Read the model definition and answer for the solid it produces. Units are mm, in the model's axes. A direction names the side the tool comes from. Give positions to 0.01 mm unless a question says otherwise; leave off trailing zeros. Write each loop counter-clockwise with the first axis right and the second up, starting at its lowest first coordinate (ties: lowest second). Pieces come first, ordered by that corner, then holes. Notation, with made-up numbers: M 85,-28 L 143,-28 A8 ccw 143,-15 Z; hole C 48,55.5 d8. An arc over 180 degrees is marked long. Use a Markdown table: item, result. Add a question column.
Item 1: For faces 4 (the cylindrical face through (9.734, -34.836, -23.778)), 5 (the flat face through (15.24, 3.4, -0.2)), 6 (the flat face through (9, -21, -38.1)), determine the directions among +Z, -Z, +X, -X, +Y, -Y from which every point of the face is accessible in a straight line to the end or side of a thin tool.
Item 2: A cutting plane is placed at B-B on x = 16.25. Determine the outline of the cut face in (y, z) (3 decimals).
Item 3: Consider probe 1 along Y at (x, z) = (11.5, 0) (1 decimal); probe 2 along X at (y, z) = (-37.25, -25.4); probe 3 along X at (y, z) = (8, -16.5). Determine where each line is inside the solid, lowest interval first. Write a range as [from, to].
Item 4: The mould has two halves that part along Y. Classify faces 1 (the cylindrical face through (8.652, -34.836, 23.587)), 2 (the cylindrical face through (8.77, -33.11, -0.24)), 3 (the conical face through (8.959, -27.667, -25.09)): pulls with the +Y half, pulls with the -Y half, needs draft (parallel to the pull), parting line crosses it, or undercut.
Item 5: Given P1, Ø8.5, axis at y = -1.5, z = -1.5, coming from the -X side; P2, Ø3, axis at y = 34.925, z = 0, coming from the +X side; P3, Ø10, axis at x = 12.5, z = -25, coming from the +Y side; P4, Ø15, axis at y = -4.5, z = -9.5, coming from the -X side, each flat-ended and moving along its own axis, determine where each tip first touches the part or whether it passes through.
Item 6: A cutting plane is placed at C-C on y = -31. Determine the outline of the cut face in (x, z), then the cut area to 3 significant figures.
Item 7: A cutting plane is placed at A-A on z = 0. Determine the outline of the cut face in (x, y) (1 decimal).
Item 8: A cutting plane is placed at D-D on y = -8. Determine the outline of the cut face in (x, z).
from build123d import *

# Parameters (mm, degrees)
SKETCH1_R                 = 38.1
BOSS_EXTRUDE1_DEPTH       = 17.78
SKETCH2_R                 = 25.4
CUT_EXTRUDE1_DEPTH        = 8.89
F_6_CLEARANCE_HOLE1_D     = 3.6576
SKETCH6_R                 = 14.2875
CUT_EXTRUDE2_DEPTH        = 6.35
SKETCH7_R                 = 3.175
CUT_EXTRUDE3_DEPTH        = 59.918282604
F_6_CLEARANCE_HOLE2_D     = 3.6576
F_6_CLEARANCE_HOLE2_DEPTH = 12.7
F_6_CLEARANCE_HOLE2_TIP   = 1.0988539


with BuildPart() as part:
    # Sketch1 → Boss-Extrude1 (new body)
    with BuildSketch(Plane(origin=(0, 0, 0), x_dir=(0, 0, -1), z_dir=(1, 0, 0))):
        with BuildLine():
            ThreePointArc((38.1, 0), (0, -38.1), (-38.1, 0))
            Line((-38.1, 0), (-38.1, -41.275))
            Line((-38.1, -41.275), (38.1, -41.275))
            Line((38.1, -41.275), (38.1, 0))
        make_face()
        Circle(SKETCH1_R)
    extrude(amount=BOSS_EXTRUDE1_DEPTH)

    # Sketch2 → Cut-Extrude1 (cut)
    with BuildSketch(Plane.ZY):
        Circle(SKETCH2_R)
    extrude(amount=-CUT_EXTRUDE1_DEPTH, mode=Mode.SUBTRACT)

    # #6 Clearance Hole1 (through all)
    with Locations(Plane(origin=(17.78, 0, 0), x_dir=(0, 0, -1), z_dir=(1, 0, 0))):
        with Locations((0, 34.925), (34.925, 0), (0, -34.925), (-34.925, 0)):
            Hole(F_6_CLEARANCE_HOLE1_D / 2)

    # Sketch6 → Cut-Extrude2 (cut)
    with BuildSketch(Plane.ZY.offset(-8.89)):
        Circle(SKETCH6_R)
    extrude(amount=-CUT_EXTRUDE2_DEPTH, mode=Mode.SUBTRACT)

    # Sketch7 → Cut-Extrude3 (cut, through all)
    with BuildSketch(Plane(origin=(17.78, 0, 0), x_dir=(0, 0, -1), z_dir=(1, 0, 0))):
        Circle(SKETCH7_R)
    extrude(amount=-CUT_EXTRUDE3_DEPTH, mode=Mode.SUBTRACT)

    # #6 Clearance Hole2
    with Locations(Plane(origin=(0, -41.275, 0), x_dir=(-1, 0, 0), z_dir=(0, -1, 0))):
        with Locations((-8.89, 25.4), (-8.89, -25.4)):
            Hole(F_6_CLEARANCE_HOLE2_D / 2, depth=F_6_CLEARANCE_HOLE2_DEPTH)
            with Locations((0, 0, -(F_6_CLEARANCE_HOLE2_DEPTH + F_6_CLEARANCE_HOLE2_TIP / 2))):  # 118° drill point
                Cone(0, F_6_CLEARANCE_HOLE2_D / 2, F_6_CLEARANCE_HOLE2_TIP, mode=Mode.SUBTRACT)


solid = part.part
Filled in:
| question | item | result |
|---|---|---|
| 1 | face 4 | -Y |
| 1 | face 5 | -X |
| 1 | face 6 | -Z, +X, -X, +Y, -Y |
| 2 | outline | M -41.275,-38.1 L 0,-38.1 A38.1 ccw 0,38.1 L -41.275,38.1 Z; hole C -34.925,0 d3.658; hole C 0,0 d6.35; hole C 0,-34.925 d3.658; hole C 0,34.925 d3.658; hole C 34.925,0 d3.658 |
| 3 | probe 1 | [-41.3, -36.8], [-33.1, -14.3], [14.3, 33.1], [36.8, 38.1] |
| 3 | probe 2 | [0, 7.06], [10.72, 17.78] |
| 3 | probe 3 | [8.89, 17.78] |
| 4 | face 1 | needs draft |
| 4 | face 2 | undercut |
| 4 | face 3 | pulls with the -Y half |
| 5 | P1 | x = 15.24 |
| 5 | P2 | through |
| 5 | P3 | y = 32.43 |
| 5 | P4 | x = 8.89 |
| 6 | outline | M 0,-38.1 L 17.78,-38.1 L 17.78,38.1 L 0,38.1 Z; hole C 8.89,-25.4 d3.66; hole C 8.89,25.4 d3.66 |
| 6 | area | 1,330 mm² |
| 7 | outline | M 0,-41.3 L 17.8,-41.3 L 17.8,-36.8 L 0,-36.8 Z; M 0,-33.1 L 17.8,-33.1 L 17.8,-3.2 L 15.2,-3.2 L 15.2,-14.3 L 8.9,-14.3 L 8.9,-25.4 L 0,-25.4 Z; M 0,25.4 L 8.9,25.4 L 8.9,14.3 L 15.2,14.3 L 15.2,3.2 L 17.8,3.2 L 17.8,33.1 L 0,33.1 Z; M 0,36.8 L 17.8,36.8 L 17.8,38.1 L 0,38.1 Z |
| 8 | outline | M 0,-38.1 L 17.78,-38.1 L 17.78,38.1 L 0,38.1 L 0,24.11 L 8.89,24.11 L 8.89,11.84 L 15.24,11.84 L 15.24,-11.84 L 8.89,-11.84 L 8.89,-24.11 L 0,-24.11 Z |
